Geometry: final body of the model. Coordinates: model frame, mm. A direction names the side the tool comes from. Coordinates: 2 decimals unless noted, no trailing zeros. Order: outer loops, then holes, each group sorted by start corner. A loop starts at its lowest first (then second) coordinate and runs counter-clockwise, first axis right, second up. Notation, with made-up numbers: (24, 50.25) -> (40, 50.25) arc R32 ccw to (40, 89.25) -> close; hole circle Ø8 at (-32.75, 14). An arc over 180 degrees is marked (long way). Answer in a Markdown table with one row per item. Add a question column.
1) Section query A-A on x = 20. Return the cut outline in (y, z), then the cut area to 3 significant figures.
2) Pull-direction query (Y, two-part tool) for faces 4 (the face through (-33.239, 45.733, 5.07)), 5 (the face through (-19.297, -42.595, 4.93)), 6 (the face through (0, -50, 5)), 7 (the face through (0, 0, 10)); classes: +Y half, -Y half, draft (parallel to the pull), parting line (faces both ways), or undercut.
3) Set-up query: faces 1 (the face through (0, 50, 5)), 2 (the face through (3.75, -38.4, 5.07)), 3 (the face through (-3.832, 38.498, 5.07)). Return all of +Z, -Z, +X, -X, +Y, -Y with unobstructed straight access to the full face (end or side cutting, diameter ignored); none if empty.
4) Section query D-D on x = 9. Return the cut outline in (y, z), then the cut area to 3 significant figures.
5) Section query C-C on y = 13. Return the cut outline in (x, z), then the cut area to 3 significant figures.
6) Section query B-B on z = 5. Return the cut outline in (x, y), then the cut area to 3 significant figures.
7) Contact query for flat-ended pins moving along their axis: P1, Ø5, axis at y = -0.5, z = 2.5, coming from the -X side; P2, Ø3, axis at y = 29, z = 5.5, coming from the +X side; P3, Ø1.5, axis at y = -24.5, z = 9, coming from the -X side. Output: stop coordinate, or through.
8) Ray query, line 1 (Y direction, x = 26, z = 1.25); line 2 (Y direction, x = -30, z = 1.5); line 3 (X direction, y = 1, z = 6). Return the intervals inside material, ascending. Write a range as from..to.
```python
from build123d import *

# Parameters (mm, degrees)
EXTRUDE_1_DEPTH = 10
FILLET_1_R      = 3.3
FILLET_2_R      = 6.5


with BuildPart() as part:
    # 草图1 → 凸台-拉伸1 (new body)
    with BuildSketch(Plane.XY):
        Polygon((34, 50), (-34, 50), (-34, 45.045833333), (-2.25, 39.754166667), (-2.25, -39.754166667), (-34, -45.045833333), (-34, -50), (34, -50), (34, -45.045833333), (2.25, -39.754166667), (2.25, 39.754166667), (34, 45.045833333), align=None)
    extrude(amount=EXTRUDE_1_DEPTH)

    # 圆角1
    fillet_1_edges = [part.edges().sort_by_distance(p)[0] for p in [
        (-34, -45.045833333, 5),
        (-34, 45.045833333, 5),
        (34, 45.045833333, 5),
        (34, -45.045833333, 5),
    ]]
    fillet(fillet_1_edges, radius=FILLET_1_R)

    # 圆角2
    fillet_2_edges = [part.edges().sort_by_distance(p)[0] for p in [
        (-2.25, -39.754166667, 5),
        (-2.25, 39.754166667, 5),
        (2.25, 39.754166667, 5),
        (2.25, -39.754166667, 5),
    ]]
    fillet(fillet_2_edges, radius=FILLET_2_R)


solid = part.part
```
Result:
| question | item | result |
|---|---|---|
| 1 | outline | (-50, 0) -> (-42.71, 0) -> (-42.71, 10) -> (-50, 10) -> close; (42.71, 0) -> (50, 0) -> (50, 10) -> (42.71, 10) -> close |
| 1 | area | 146 mm2 |
| 2 | face 4 | undercut |
| 2 | face 5 | undercut |
| 2 | face 6 | -Y half |
| 2 | face 7 | draft |
| 3 | face 1 | +Z, -Z, +X, -X, +Y |
| 3 | face 2 | +Z, -Z, +X |
| 3 | face 3 | +Z, -Z, -X |
| 4 | outline | (-50, 0) -> (-40.88, 0) -> (-40.88, 10) -> (-50, 10) -> close; (40.88, 0) -> (50, 0) -> (50, 10) -> (40.88, 10) -> close |
| 4 | area | 182 mm2 |
| 5 | outline | (-2.25, 0) -> (2.25, 0) -> (2.25, 10) -> (-2.25, 10) -> close |
| 5 | area | 45.0 mm2 |
| 6 | outline | (-34, -50) -> (34, -50) -> (34, -47.84) arc R3.3 ccw to (31.24, -44.59) -> (7.68, -40.66) arc R6.5 cw to (2.25, -34.25) -> (2.25, 34.25) arc R6.5 cw to (7.68, 40.66) -> (31.24, 44.59) arc R3.3 ccw to (34, 47.84) -> (34, 50) -> (-34, 50) -> (-34, 47.84) arc R3.3 ccw to (-31.24, 44.59) -> (-7.68, 40.66) arc R6.5 cw to (-2.25, 34.25) -> (-2.25, -34.25) arc R6.5 cw to (-7.68, -40.66) -> (-31.24, -44.59) arc R3.3 ccw to (-34, -47.84) -> close |
| 6 | area | 1,430 mm2 |
| 7 | P1 | x = -2.25 |
| 7 | P2 | x = 2.25 |
| 7 | P3 | x = -2.25 |
| 8 | line 1 | -50..-43.71, 43.71..50 |
| 8 | line 2 | -50..-44.38, 44.38..50 |
| 8 | line 3 | -2.25..2.25 |
